Answer from the drawing. Dimensions are ordinates in mm from the lowest x, y and z of the part. Coordinates: 2 decimals unless noted, no trailing zeros. Write each loop counter-clockwise with the first axis right and the second up, starting at its lowest first coordinate (ties: lowest second). Pieces come first, ordered by that corner, then holes.
(1) The part is cut by section B-B on x = 129. Determine the outline of the cut face in (y, z).
(2) Straight lines are drawn through the part: line 1 (Y direction, x = 37, z = 1.75); line 2 (X direction, y = 65, z = 6). For each, find the intervals that lie inside material, in ascending order.
(3) Given P1, Ø3, axis at x = 121, z = 7, coming from the +Y side; P2, Ø4, axis at x = 74.5, z = 6, coming from the -Y side; P3, Ø3, axis at x = 4, z = 6.5, coming from the -Y side; P4, Ø5, axis at y = 3.5, z = 5.5, coming from the +X side, each flat-ended and moving along its own axis, determine where each tip first touches the part or whether it passes through.
(4) The part is cut by section A-A on y = 37. Determine the outline of the cut face in (x, z).
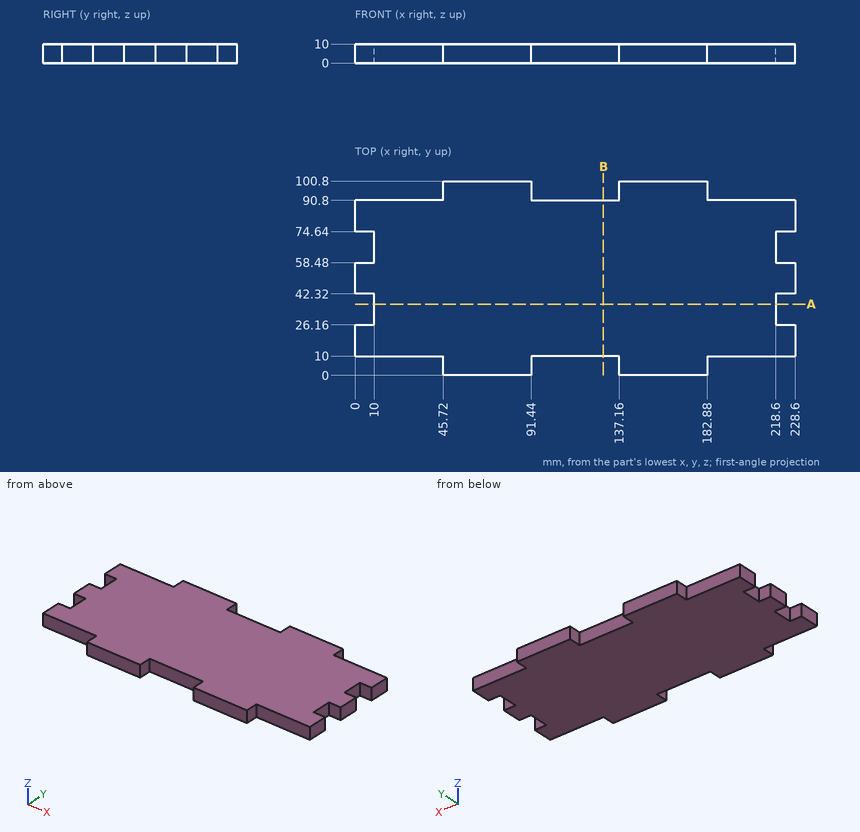
Model answer:
1. outline: (10, 0) - (90.8, 0) - (90.8, 10) - (10, 10) - close
2. line 1: y = 10 to 90.8
2. line 2: x = 10 to 218.6
3. P1: stops at y = 90.8
3. P2: stops at y = 0
3. P3: stops at y = 10
3. P4: stops at x = 182.88
4. outline: (10, 0) - (218.6, 0) - (218.6, 10) - (10, 10) - close
